For this review, take the finished solid that the model builds, in its own axes (mm). Face numbers are marked on the shaded views. A direction names the side the tool comes from. Give positions to 0.01 mm unless a question says otherwise; leave off trailing zeros. Order: outer loops, then holes, each group sorted by start corner. A loop starts at its lowest first (then second) coordinate and runs counter-clockwise, first axis right, second up. Notation, with made-up numbers: M 49,64.5 L 91,64.5 A23 cw 91,83.5 Z; hole C -5,-0.5 d4. An arc over 180 degrees is marked long. Answer as CSV lines item,"result". Start each with the question number.
1. For line 1 along Y through (x, z) = (-2.5, -0.25) (3 decimals); line 2 along X through (y, z) = (1.75, 0); line 3 along Y through (x, z) = (2, -2.5) (3 decimals), list the stretches that pass through material, from the lowest coordinate up.
2. We need section A-A, the plane y = 9.75. Give the boundary of the cut face in (x, z), and give its area (3 significant figures).
3. We need section B-B, the plane y = 4.5. Give the boundary of the cut face in (x, z).
4. Machinability: for the marked faces 1 and 2, which of the approach directions +Z, -Z, +X, -X, +Y, -Y give a long, thin tool a straight path to every point of the face, cutting with its end or side? Answer none if there is none.
5. Clearance check with flat-ended pins moving along their axes: P1, Ø2, axis at x = -4, z = 4, coming from the -Y side (3 decimals); P2, Ø0.8, axis at y = 12, z = 2, coming from the +X side; P3, Ø1.5, axis at y = 2.5, z = 3.5, coming from the -X side; P4, Ø4, axis at y = 11, z = -2.5, coming from the +X side. State where each tip first meets the part, or that it passes through.
6. Mouldability with a two-part tool opening along X and no side actions: class the marked faces 3, 4 and 5 as pulls with the +X half, pulls with the -X half, needs draft (parallel to the pull), parting line crosses it, or undercut.
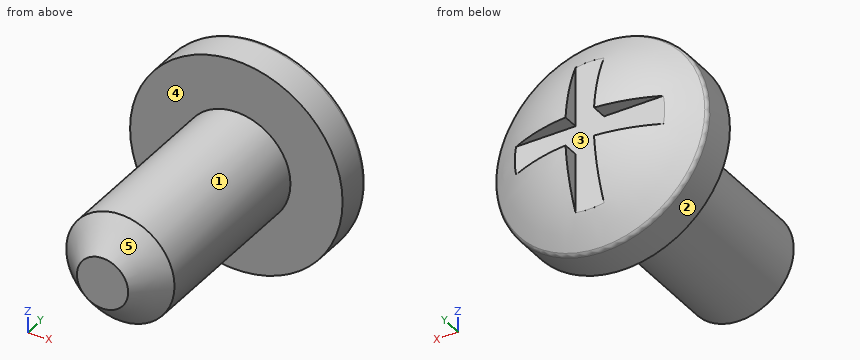
from build123d import *

# Parameters (mm, degrees)
CUT_EXTRUDE1_DEPTH = 0.635
CIRPATTERN1_COUNT  = 4
CHAMFER1_SIZE      = 1.27
FILLET1_R          = 0.254


with BuildPart() as part:
    # Sketch1 → Revolve1 (revolve)
    with BuildSketch(Plane.XY):
        with BuildLine():
            Line((0, 0), (2.413, 0))
            Line((2.413, 0), (2.413, 9.525))
            Line((2.413, 9.525), (4.7371, 9.525))
            Line((4.7371, 9.525), (4.7371, 11.076185676))
            ThreePointArc((4.7371, 11.076185676), (2.503841517, 12.282774321), (0, 12.7))
            Line((0, 12.7), (0, 0))
        make_face()
    revolve(axis=Axis((0, 0, 0), (0, 1, 0)))

    # Sketch2 → Cut-Extrude1 (cut, symmetric)
    with BuildSketch(Plane.XY):
        with BuildLine():
            Line((0, 12.7), (0, 11.938))
            Line((0, 11.938), (3.344708418, 11.938))
            ThreePointArc((3.344708418, 11.938), (1.71520541, 12.507090255), (0, 12.7))
        make_face()
    cut_extrude1 = extrude(amount=CUT_EXTRUDE1_DEPTH, both=True, mode=Mode.SUBTRACT)

    # CirPattern1: Cut-Extrude1 ×4 about axis
    cirpattern1_axis = Axis((0, 0, 0), (0, 1, 0))
    for i in range(1, CIRPATTERN1_COUNT):
        add(cut_extrude1.rotate(cirpattern1_axis, i * 360 / CIRPATTERN1_COUNT), mode=Mode.SUBTRACT)

    # Chamfer1
    chamfer1_edges = [part.edges().sort_by_distance(p)[0] for p in [
        (-2.413, 0, 0),
    ]]
    chamfer(chamfer1_edges, length=CHAMFER1_SIZE)

    # Fillet1
    fillet1_edges = [part.edges().sort_by_distance(p)[0] for p in [
        (-4.7371, 11.076185676, 0),
    ]]
    fillet(fillet1_edges, radius=FILLET1_R)


solid = part.part
Result set:
1,line 1,"9.525 to 11.938"
1,line 2,"-2.41 to 2.41"
1,line 3,"9.525 to 12.005"
2,outline,"C 0,0 d9.47"
2,area,"70.5 mm2"
3,outline,"C 0,0 d4.83"
4,face 1,"-Y"
4,face 2,"+Y, -Y"
5,P1,"y = 9.525"
5,P2,"x = 3.46"
5,P3,"through"
5,P4,"x = 4.71"
6,face 3,"undercut"
6,face 4,"needs draft"
6,face 5,"parting line crosses it"
